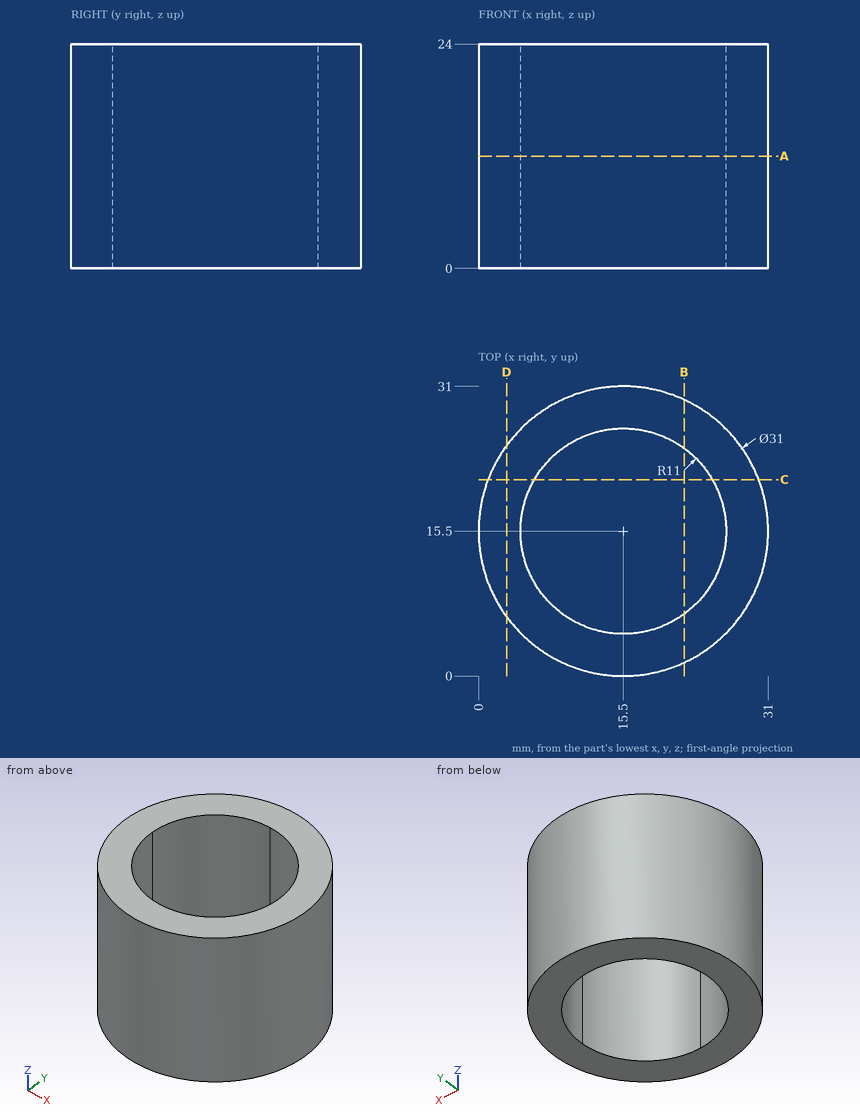
Geometry: see drawing. Coordinates: mm, zero at the bounding-box minimum. Coordinates: 2 decimals unless noted, no trailing zeros. Loops run counter-clockwise (first coordinate to the right, second up) from the corner with the lowest first, then second, coordinate; pieces in that order, holes last. Notation, with made-up numbers: M -11,72.25 L 21,72.25 A14 ccw 21,88.25 Z; hole C 73,-18.5 d4. An arc over 180 degrees is marked long. Put each result on its own line as item: value. Start each with the question number.
1) Contact query for flat-ended pins moving along their axis: pin 1 Ø1.5 at (y, z) = (25.5, 4.5) entering from -X; pin 2 Ø6 at (y, z) = (25, 14.5) entering from -X; pin 3 Ø8 at (x, z) = (25, 19.5) entering from -Y. Output: stop coordinate, or through.
2) Cut plane D-D on x = 3. Return the cut outline in (y, z), then the cut area to 3 significant figures.
3) Cut plane B-B on x = 22. Return the cut outline in (y, z), then the cut area to 3 significant figures.
4) Cut plane A-A on z = 12. Return the cut outline in (x, y).
5) Cut plane C-C on y = 21. Return the cut outline in (x, z).
6) Ray query, L1, parallel to X at y = 20, z = 19.25; L2, parallel to Y at x = 6, z = 2.75; L3, parallel to Y at x = 24.5, z = 3.75. Return the intervals inside material, ascending. Write a range as from..to.
The answers:
1. pin 1: stops at x = 3.06
1. pin 2: stops at x = 1.43
1. pin 3: stops at y = 1.01
2. outline: M 6.33,0 L 24.67,0 L 24.67,24 L 6.33,24 Z
2. area: 440 mm²
3. outline: M 1.43,0 L 6.63,0 L 6.63,24 L 1.43,24 Z; M 24.37,0 L 29.57,0 L 29.57,24 L 24.37,24 Z
3. area: 249 mm²
4. outline: C 15.5,15.5 d31; hole C 15.5,15.5 d22
5. outline: M 1.01,0 L 5.97,0 L 5.97,24 L 1.01,24 Z; M 25.03,0 L 29.99,0 L 29.99,24 L 25.03,24 Z
6. L1: x = 0.67..5.46, 25.54..30.33
6. L2: y = 3.25..9.95, 21.05..27.75
6. L3: y = 2.88..9.18, 21.82..28.12
